For this review, take the finished solid that the model builds, in its own axes (mm). Face numbers are marked on the shaded views. A direction names the side the tool comes from. Round coordinates to 2 decimals unless told otherwise and drop trailing zeros. Order: outer loops, then holes, each group sorted by start corner. A loop starts at its lowest first (then second) coordinate and runs counter-clockwise, first axis right, second up. Notation, with made-up numbers: (62, -21) -> (71, -21) arc R11 ccw to (71, -14) -> close; hole circle Ø5 at (-1.5, 70). An arc over 180 degrees is marked (long way). Use a Markdown table: item, result. Add a question column.
1) Consider section A-A (x = 21). State the section outline as (y, z) points, plus the area to 3 significant figures.
2) Consider section C-C (x = 14). State the section outline as (y, z) points.
3) Clearance check with flat-ended pins moving along their axes: P1, Ø5, axis at y = -3.5, z = 19, coming from the +X side; P2, Ø9.5, axis at x = 28, y = 1.5, coming from the +Z side. State where each tip first meets the part, or that it passes through.
4) Machinability: for the marked faces 1 and 2, which of the approach directions +Z, -Z, +X, -X, +Y, -Y give a long, thin tool a straight path to every point of the face, cutting with its end or side? Answer none if there is none.
5) Consider section D-D (z = 4.5). State the section outline as (x, y) points, plus the area to 3 significant figures.
6) Wall thickness on line 1 along X through (y, z) = (-19, 28.5); line 2 along Z through (x, y) = (33, 20); line 3 along Y through (x, z) = (16, 6.5): over which ranges is each line inside the solid? List them lowest first. Write a range as [from, to].
7) Consider section B-B (y = 32). State the section outline as (x, z) points, plus the area to 3 significant figures.
8) Draft analysis for pull direction X (two halves, no side actions). For the marked faces 3, 4 and 5, state which applies: pulls with the +X half, pulls with the -X half, needs draft (parallel to the pull), parting line crosses it, or undercut.
```python
from build123d import *

# Parameters (mm, degrees)
F1_DEPTH = 50.8
F2_R     = 7.1318057121
F3_DEPTH = 25.4


with BuildPart() as f1:
    # F0 (on Front) → F1 (new body, symmetric)
    with BuildSketch(Plane.XZ):
        Polygon((0, 35.6939397752), (0, 0), (36.6625972092, 0), (36.6625972092, 6.5840519965), (5.6025939994, 6.5840519965), (5.6025939994, 35.6939397752), align=None)
    extrude(amount=F1_DEPTH, both=True)

    # F2 (on face) → F3 (cut)
    with BuildSketch(Plane.XY.offset(6.5840519965)):
        with Locations((18.8083481044, -12.6618258655)):
            Circle(F2_R)
    extrude(amount=-F3_DEPTH, mode=Mode.SUBTRACT)


solid = f1.part
```
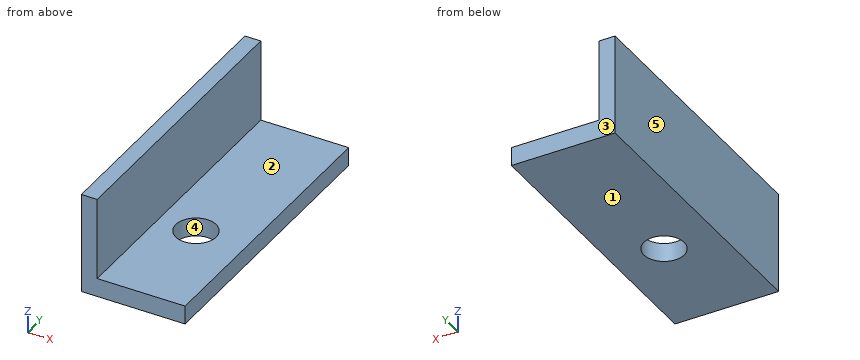
Results list:
| question | item | result |
|---|---|---|
| 1 | outline | (-50.8, 0) -> (-19.45, 0) -> (-19.45, 6.58) -> (-50.8, 6.58) -> close; (-5.88, 0) -> (50.8, 0) -> (50.8, 6.58) -> (-5.88, 6.58) -> close |
| 1 | area | 580 mm2 |
| 2 | outline | (-50.8, 0) -> (-17.93, 0) -> (-17.93, 6.58) -> (-50.8, 6.58) -> close; (-7.39, 0) -> (50.8, 0) -> (50.8, 6.58) -> (-7.39, 6.58) -> close |
| 3 | P1 | x = 5.6 |
| 3 | P2 | z = 6.58 |
| 4 | face 1 | -Z, +X, -X, +Y, -Y |
| 4 | face 2 | +Z, +X, +Y, -Y |
| 5 | outline | (0, -50.8) -> (36.66, -50.8) -> (36.66, 50.8) -> (0, 50.8) -> close; hole circle Ø14.26 at (18.81, -12.66) |
| 5 | area | 3,570 mm2 |
| 6 | line 1 | [0, 5.6] |
| 6 | line 2 | [0, 6.58] |
| 6 | line 3 | [-50.8, -19.22], [-6.11, 50.8] |
| 7 | outline | (0, 0) -> (36.66, 0) -> (36.66, 6.58) -> (5.6, 6.58) -> (5.6, 35.69) -> (0, 35.69) -> close |
| 7 | area | 404 mm2 |
| 8 | face 3 | needs draft |
| 8 | face 4 | undercut |
| 8 | face 5 | pulls with the -X half |
